from build123d import *

# Parameters (mm, degrees)
SKETCH1_W                = 210
SKETCH1_H                = 70
BOSS_EXTRUDE1_DEPTH      = 3
SKETCH2_W                = 10
SKETCH2_H                = 3
CUT_EXTRUDE1_DEPTH       = 3
LPATTERN1_COUNT          = 11
LPATTERN1_PITCH          = 20
MIRROR1_COPY_1_SKETCH_W  = 10
MIRROR1_COPY_1_SKETCH_H  = 3
MIRROR1_COPY_1_DEPTH     = 3
MIRROR1_COPY_2_SKETCH_W  = 10
MIRROR1_COPY_2_SKETCH_H  = 3
MIRROR1_COPY_2_DEPTH     = 3
MIRROR1_COPY_3_SKETCH_W  = 10
MIRROR1_COPY_3_SKETCH_H  = 3
MIRROR1_COPY_3_DEPTH     = 3
MIRROR1_COPY_4_SKETCH_W  = 10
MIRROR1_COPY_4_SKETCH_H  = 3
MIRROR1_COPY_4_DEPTH     = 3
MIRROR1_COPY_5_SKETCH_W  = 10
MIRROR1_COPY_5_SKETCH_H  = 3
MIRROR1_COPY_5_DEPTH     = 3
MIRROR1_COPY_6_SKETCH_W  = 10
MIRROR1_COPY_6_SKETCH_H  = 3
MIRROR1_COPY_6_DEPTH     = 3
MIRROR1_COPY_7_SKETCH_W  = 10
MIRROR1_COPY_7_SKETCH_H  = 3
MIRROR1_COPY_7_DEPTH     = 3
MIRROR1_COPY_8_SKETCH_W  = 10
MIRROR1_COPY_8_SKETCH_H  = 3
MIRROR1_COPY_8_DEPTH     = 3
MIRROR1_COPY_9_SKETCH_W  = 10
MIRROR1_COPY_9_SKETCH_H  = 3
MIRROR1_COPY_9_DEPTH     = 3
MIRROR1_COPY_10_SKETCH_W = 10
MIRROR1_COPY_10_SKETCH_H = 3
MIRROR1_COPY_10_DEPTH    = 3
SKETCH3_W                = 3
SKETCH3_H                = 10
CUT_EXTRUDE2_DEPTH       = 3
LPATTERN2_COUNT          = 3
LPATTERN2_PITCH          = 20
MIRROR2_COPY_1_SKETCH_W  = 3
MIRROR2_COPY_1_SKETCH_H  = 10
MIRROR2_COPY_1_DEPTH     = 3
MIRROR2_COPY_2_SKETCH_W  = 3
MIRROR2_COPY_2_SKETCH_H  = 10
MIRROR2_COPY_2_DEPTH     = 3
SKETCH4_W                = 6
SKETCH4_H                = 50
CUT_EXTRUDE3_DEPTH       = 3
LPATTERN3_COUNT          = 10
LPATTERN3_PITCH          = 20


with BuildPart() as part:
    # Sketch1 → Boss-Extrude1 (new body)
    with BuildSketch(Plane(origin=(0, 0, 0), x_dir=(0, 0, -1), z_dir=(1, 0, 0))):
        Rectangle(SKETCH1_W, SKETCH1_H)
    extrude(amount=BOSS_EXTRUDE1_DEPTH)

    # Sketch2 → Cut-Extrude1 (cut)
    with BuildSketch(Plane(origin=(3, 0, 0), x_dir=(0, 0, -1), z_dir=(1, 0, 0))):
        with Locations((-100, 33.5)):
            Rectangle(SKETCH2_W, SKETCH2_H)
    cut_extrude1 = extrude(amount=-CUT_EXTRUDE1_DEPTH, mode=Mode.SUBTRACT)

    # LPattern1: Cut-Extrude1 ×11
    with Locations(*[(0, 0, -i * LPATTERN1_PITCH) for i in range(1, LPATTERN1_COUNT)]):
        add(cut_extrude1, mode=Mode.SUBTRACT)

    # Mirror1: Cut-Extrude1 across plane
    add(cut_extrude1.mirror(Plane.ZX), mode=Mode.SUBTRACT)

    # Mirror1 copy 1 sketch → Mirror1 copy 1 (cut)
    with BuildSketch(Plane(origin=(3, 0, -20), x_dir=(0, 0, -1), z_dir=(1, 0, 0))):
        with Locations((-100, -33.5)):
            Rectangle(MIRROR1_COPY_1_SKETCH_W, MIRROR1_COPY_1_SKETCH_H)
    extrude(amount=-MIRROR1_COPY_1_DEPTH, mode=Mode.SUBTRACT)

    # Mirror1 copy 2 sketch → Mirror1 copy 2 (cut)
    with BuildSketch(Plane(origin=(3, 0, -40), x_dir=(0, 0, -1), z_dir=(1, 0, 0))):
        with Locations((-100, -33.5)):
            Rectangle(MIRROR1_COPY_2_SKETCH_W, MIRROR1_COPY_2_SKETCH_H)
    extrude(amount=-MIRROR1_COPY_2_DEPTH, mode=Mode.SUBTRACT)

    # Mirror1 copy 3 sketch → Mirror1 copy 3 (cut)
    with BuildSketch(Plane(origin=(3, 0, -60), x_dir=(0, 0, -1), z_dir=(1, 0, 0))):
        with Locations((-100, -33.5)):
            Rectangle(MIRROR1_COPY_3_SKETCH_W, MIRROR1_COPY_3_SKETCH_H)
    extrude(amount=-MIRROR1_COPY_3_DEPTH, mode=Mode.SUBTRACT)

    # Mirror1 copy 4 sketch → Mirror1 copy 4 (cut)
    with BuildSketch(Plane(origin=(3, 0, -80), x_dir=(0, 0, -1), z_dir=(1, 0, 0))):
        with Locations((-100, -33.5)):
            Rectangle(MIRROR1_COPY_4_SKETCH_W, MIRROR1_COPY_4_SKETCH_H)
    extrude(amount=-MIRROR1_COPY_4_DEPTH, mode=Mode.SUBTRACT)

    # Mirror1 copy 5 sketch → Mirror1 copy 5 (cut)
    with BuildSketch(Plane(origin=(3, 0, -100), x_dir=(0, 0, -1), z_dir=(1, 0, 0))):
        with Locations((-100, -33.5)):
            Rectangle(MIRROR1_COPY_5_SKETCH_W, MIRROR1_COPY_5_SKETCH_H)
    extrude(amount=-MIRROR1_COPY_5_DEPTH, mode=Mode.SUBTRACT)

    # Mirror1 copy 6 sketch → Mirror1 copy 6 (cut)
    with BuildSketch(Plane(origin=(3, 0, -120), x_dir=(0, 0, -1), z_dir=(1, 0, 0))):
        with Locations((-100, -33.5)):
            Rectangle(MIRROR1_COPY_6_SKETCH_W, MIRROR1_COPY_6_SKETCH_H)
    extrude(amount=-MIRROR1_COPY_6_DEPTH, mode=Mode.SUBTRACT)

    # Mirror1 copy 7 sketch → Mirror1 copy 7 (cut)
    with BuildSketch(Plane(origin=(3, 0, -140), x_dir=(0, 0, -1), z_dir=(1, 0, 0))):
        with Locations((-100, -33.5)):
            Rectangle(MIRROR1_COPY_7_SKETCH_W, MIRROR1_COPY_7_SKETCH_H)
    extrude(amount=-MIRROR1_COPY_7_DEPTH, mode=Mode.SUBTRACT)

    # Mirror1 copy 8 sketch → Mirror1 copy 8 (cut)
    with BuildSketch(Plane(origin=(3, 0, -160), x_dir=(0, 0, -1), z_dir=(1, 0, 0))):
        with Locations((-100, -33.5)):
            Rectangle(MIRROR1_COPY_8_SKETCH_W, MIRROR1_COPY_8_SKETCH_H)
    extrude(amount=-MIRROR1_COPY_8_DEPTH, mode=Mode.SUBTRACT)

    # Mirror1 copy 9 sketch → Mirror1 copy 9 (cut)
    with BuildSketch(Plane(origin=(3, 0, -180), x_dir=(0, 0, -1), z_dir=(1, 0, 0))):
        with Locations((-100, -33.5)):
            Rectangle(MIRROR1_COPY_9_SKETCH_W, MIRROR1_COPY_9_SKETCH_H)
    extrude(amount=-MIRROR1_COPY_9_DEPTH, mode=Mode.SUBTRACT)

    # Mirror1 copy 10 sketch → Mirror1 copy 10 (cut)
    with BuildSketch(Plane(origin=(3, 0, -200), x_dir=(0, 0, -1), z_dir=(1, 0, 0))):
        with Locations((-100, -33.5)):
            Rectangle(MIRROR1_COPY_10_SKETCH_W, MIRROR1_COPY_10_SKETCH_H)
    extrude(amount=-MIRROR1_COPY_10_DEPTH, mode=Mode.SUBTRACT)

    # Sketch3 → Cut-Extrude2 (cut)
    with BuildSketch(Plane(origin=(3, 0, 0), x_dir=(0, 0, -1), z_dir=(1, 0, 0))):
        with Locations((-103.5, 20)):
            Rectangle(SKETCH3_W, SKETCH3_H)
    cut_extrude2 = extrude(amount=-CUT_EXTRUDE2_DEPTH, mode=Mode.SUBTRACT)

    # LPattern2: Cut-Extrude2 ×3
    with Locations(*[(0, -i * LPATTERN2_PITCH, 0) for i in range(1, LPATTERN2_COUNT)]):
        add(cut_extrude2, mode=Mode.SUBTRACT)

    # Mirror2: Cut-Extrude2 across plane
    add(cut_extrude2.mirror(Plane.XY), mode=Mode.SUBTRACT)

    # Mirror2 copy 1 sketch → Mirror2 copy 1 (cut)
    with BuildSketch(Plane(origin=(3, -20, 0), x_dir=(0, 0, 1), z_dir=(1, 0, 0))):
        with Locations((-103.5, -20)):
            Rectangle(MIRROR2_COPY_1_SKETCH_W, MIRROR2_COPY_1_SKETCH_H)
    extrude(amount=-MIRROR2_COPY_1_DEPTH, mode=Mode.SUBTRACT)

    # Mirror2 copy 2 sketch → Mirror2 copy 2 (cut)
    with BuildSketch(Plane(origin=(3, -40, 0), x_dir=(0, 0, 1), z_dir=(1, 0, 0))):
        with Locations((-103.5, -20)):
            Rectangle(MIRROR2_COPY_2_SKETCH_W, MIRROR2_COPY_2_SKETCH_H)
    extrude(amount=-MIRROR2_COPY_2_DEPTH, mode=Mode.SUBTRACT)

    # Sketch4 → Cut-Extrude3 (cut)
    with BuildSketch(Plane(origin=(3, 0, 0), x_dir=(0, 0, -1), z_dir=(1, 0, 0))):
        with Locations((-90, 0)):
            Rectangle(SKETCH4_W, SKETCH4_H)
    cut_extrude3 = extrude(amount=-CUT_EXTRUDE3_DEPTH, mode=Mode.SUBTRACT)

    # LPattern3: Cut-Extrude3 ×10
    with Locations(*[(0, 0, -i * LPATTERN3_PITCH) for i in range(1, LPATTERN3_COUNT)]):
        add(cut_extrude3, mode=Mode.SUBTRACT)


solid = part.part
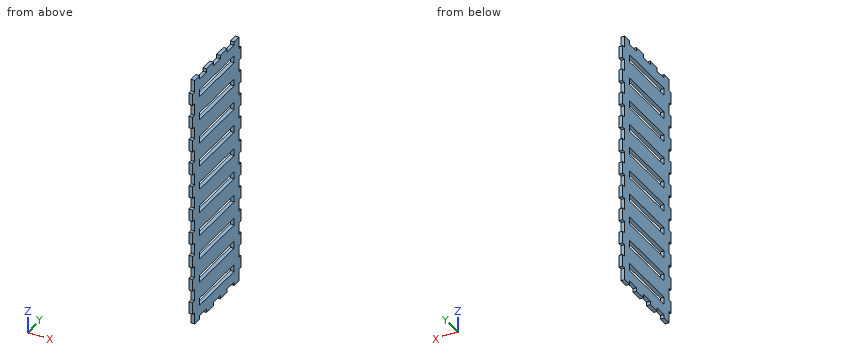
Model file for the job. Use its own axes, mm. Give positions to 0.01 mm unless a question says otherwise; leave off trailing zeros. Write each loop counter-clockwise with the first axis right and the second up, starting at its lowest first coordinate (ties: lowest second). Pieces come first, ordered by that corner, then holes. Notation, with made-up numbers: (-33, 42) - (8, 42) arc R21 cw to (8, 72) - close; hole circle Ø11 at (38.25, -34). An arc over 180 degrees is marked (long way). Answer as CSV lines item,"result".
1. Drill centre lines: L1, parallel to Y at x = 1.15, z = -31.5; L2, parallel to Y at x = 2.85, z = 77. Where is each one in solid material? Low to high. Write a range as [from, to].
Responses:
L1,"y = [-35, -25], [25, 35]"
L2,"y = [-32, 32]"
2. Band-saw the part on C-C (z = -21). Write the cut outline in (x, y).
Responses:
outline,"(0, -32) - (3, -32) - (3, 32) - (0, 32) - close"
3. Pin check, flat tips, straight feed: pin 1 (1 mm diameter, centred on x = 1, z = -42.5, fed in from +Y); pin 2 (1.5 mm diameter, centred on x = 0.5, z = 22, fed in from -Y); pin 3 (0.9 mm diameter, centred on x = 1.5, y = 33.5, fed in from -Z). Stop position of each tip, or through.
Responses:
pin 1,"stops at y = 32"
pin 2,"stops at y = -32"
pin 3,"stops at z = -95"
4. Band-saw the part on B-B (y = 10.5). Count the separate pieces of the cut face and the enclosed holes in it, and give its area (3 significant figures).
Responses:
separate pieces,"11"
enclosed holes,"0"
area,"450 mm2"
5. Band-saw the part on A-A (z = 29). Write the cut outline in (x, y), and give its area (3 significant figures).
Responses:
outline,"(0, -35) - (3, -35) - (3, -25) - (0, -25) - close; (0, 25) - (3, 25) - (3, 35) - (0, 35) - close"
area,"60.0 mm2"
